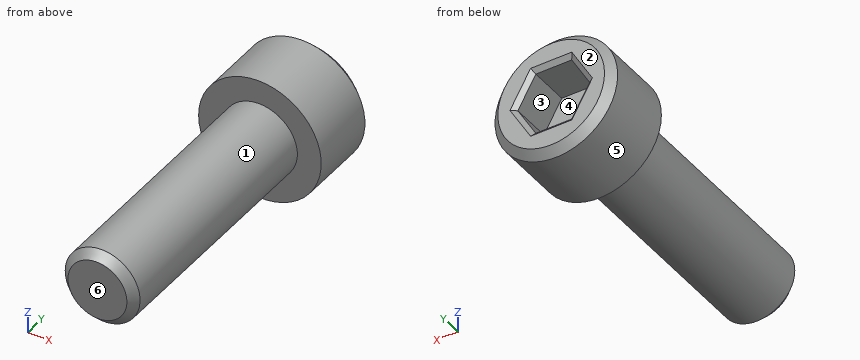
```python
from build123d import *

# Parameters (mm, degrees)
EXTRUDE1_DEPTH = 2.794
CHAMFER1_SIZE  = 0.508
CHAMFER2_SIZE  = 0.29329394
CHAMFER2_SIZE2 = 0.253999961


with BuildPart() as part:
    # Sketch1 → Revolve1 (revolve)
    with BuildSketch(Plane.XY):
        Polygon((0, 0), (0, 20.6502), (-3.9116, 20.6502), (-3.9116, 15.875), (-2.3876, 15.875), (-2.3876, 0), align=None)
    revolve(axis=Axis((0, 0, 0), (0, 1, 0)))

    # Sketch2 → Extrude1 (cut)
    with BuildSketch(Plane(origin=(0, 20.6502, 0), x_dir=(1, 0, 0), z_dir=(0, 1, 0))):
        Polygon((2.2913594, 0), (1.1456797, 1.98437545), (-1.1456797, 1.98437545), (-2.2913594, 0), (-1.1456797, -1.98437545), (1.1456797, -1.98437545), align=None)
    extrude(amount=-EXTRUDE1_DEPTH, mode=Mode.SUBTRACT)

    # Chamfer1
    chamfer1_edges = [part.edges().sort_by_distance(p)[0] for p in [
        (2.3876, 0, 0),
        (3.9116, 20.6502, 0),
    ]]
    chamfer(chamfer1_edges, length=CHAMFER1_SIZE)

    # Chamfer2
    chamfer2_edges = [part.edges().sort_by_distance(p)[0] for p in [
        (1.71851955, 20.6502, 0.992187725),
        (1.71851955, 20.6502, -0.992187725),
        (0, 20.6502, -1.98437545),
        (-1.71851955, 20.6502, -0.992187725),
        (-1.71851955, 20.6502, 0.992187725),
        (0, 20.6502, 1.98437545),
    ]]
    chamfer2_side = [part.faces().sort_by_distance(p)[0] for p in [
        (3.307331654, 20.6502, 0),
    ]]
    chamfer(chamfer2_edges, length=CHAMFER2_SIZE, length2=CHAMFER2_SIZE2, reference=chamfer2_side[0])


solid = part.part
```
Check sheet for the modelled part. Datum: model origin and axes. Units: mm. Face numbers are marked on the shaded views. A direction names the side the tool comes from. Give positions to 0.01 mm unless a question says otherwise; leave off trailing zeros. Order: outer loops, then holes, each group sorted by start corner. A loop starts at its lowest first (then second) coordinate and runs counter-clockwise, first axis right, second up. Notation, with made-up numbers: M 44.25,-15 L 78.25,-15 A15 ccw 78.25,2 Z; hole C 80,-6.75 d10. An arc over 180 degrees is marked long. Answer in a Markdown table with one row per item.
1) Release check for a two-part mould opening along Z. For the marked faces 4, 5 and 6 record: +Z half, -Z half, draft (parallel to the pull), parting line (faces both ways), or undercut.
Filled sheet:
| item | result |
|---|---|
| face 4 | undercut |
| face 5 | parting line |
| face 6 | draft |
2) Cross-section at B-B, the plane y = 17. Enter the section's corners in (x, z), plus the area to 3 significant figures.
Filled sheet:
| item | result |
|---|---|
| outline | C 0,0 d7.82 |
| area | 48.1 mm2 |
3) Thickness scan on L1, parallel to Y at x = -1, z = -1.25; L2, parallel to Y at x = 2.5, z = -2.25 (3 decimals); L3, parallel to X at y = 19, z = 1.75. Record the ranges inside material, lowest first. Write a range as [from, to].
Filled sheet:
| item | result |
|---|---|
| L1 | y = [0, 17.86] |
| L2 | y = [15.875, 20.65] |
| L3 | x = [-3.5, -1.28], [1.28, 3.5] |
4) Cross-section at C-C, the plane y = 13.5. Enter the section's corners in (x, z), plus the area to 3 significant figures.
Filled sheet:
| item | result |
|---|---|
| outline | C 0,0 d4.78 |
| area | 17.9 mm2 |
5) Access from +Z, -Z, +X, -X, +Y, -Y to the whole of each face (thin tool, end or side, straight path). Record for the marked faces 1, 2 and 3.
Filled sheet:
| item | result |
|---|---|
| face 1 | -Y |
| face 2 | +Z, -Z, +X, -X, +Y |
| face 3 | +Y |
6) Gauge pin test, flat ends, axial feed: P1, Ø1.5, axis at x = -2.5, z = 2, coming from the -Y side (3 decimals); P2, Ø1.2, axis at x = 1, z = 0.5, coming from the +Y side; P3, Ø1, axis at y = 7.5, z = 0.5, coming from the +X side. Record the tip position at first contact, or that the pin passes through.
Filled sheet:
| item | result |
|---|---|
| P1 | stops at y = 15.875 |
| P2 | stops at y = 17.86 |
| P3 | stops at x = 2.39 |
7) Cross-section at A-A, the plane x = 0. Enter the section's corners in (y, z) (3 decimals), plus the area to 3 significant figures.
Filled sheet:
| item | result |
|---|---|
| outline | M 0,-1.88 L 0.508,-2.388 L 15.875,-2.388 L 15.875,-3.912 L 20.142,-3.912 L 20.65,-3.404 L 20.65,-2.278 L 20.396,-1.984 L 17.856,-1.984 L 17.856,1.984 L 20.396,1.984 L 20.65,2.278 L 20.65,3.404 L 20.142,3.912 L 15.875,3.912 L 15.875,2.388 L 0.508,2.388 L 0,1.88 Z |
| area | 101 mm2 |
